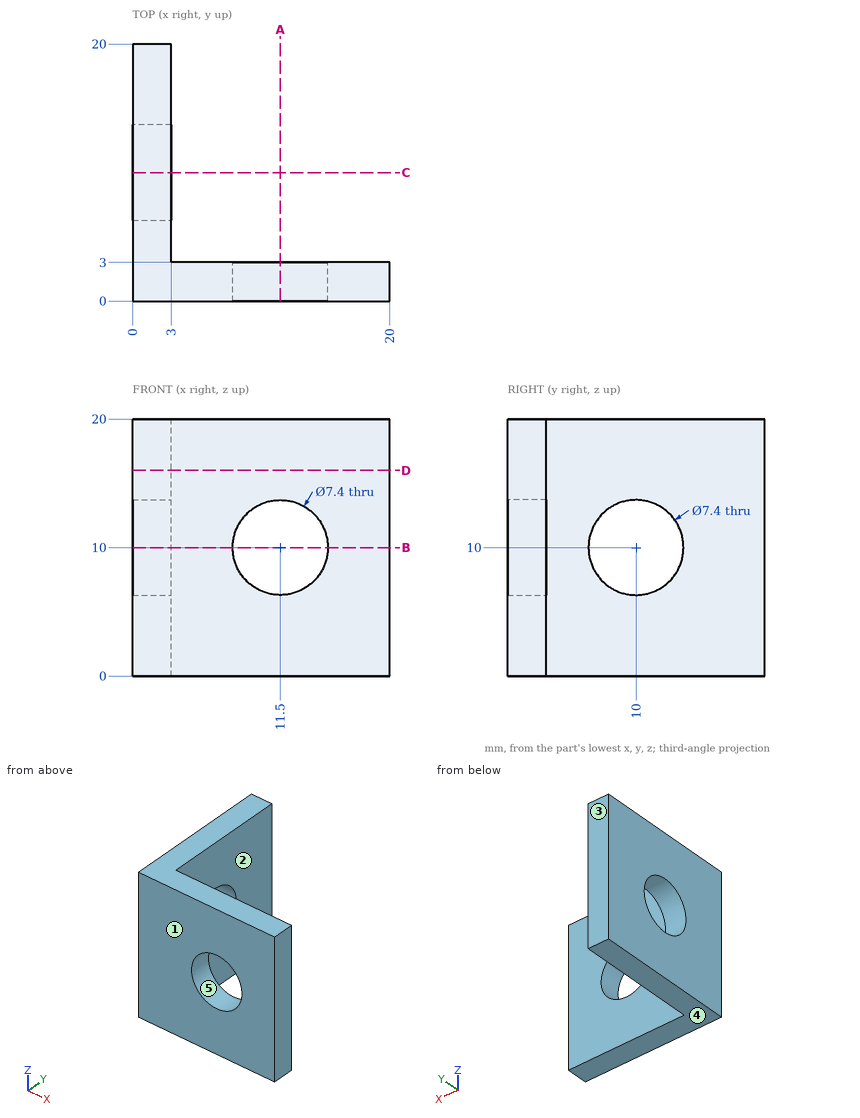
Part print with two shaded views. Sizes in mm from the minimum x, y, z corner. A direction names the side the tool comes from. Give positions to 0.01 mm unless a question says otherwise; leave off trailing zeros. Order: outer loops, then holes, each group sorted by start corner. A loop starts at its lowest first (then second) coordinate and runs counter-clockwise, first axis right, second up.
(1) Drill centre lines: L1, parallel to Z at x = 1.45, y = 10; L2, parallel to X at y = 1.75, z = 10; L3, parallel to X at y = 6.5, z = 2.25. Where is each one in solid material? Low to high.
(2) Flat gauge pins, fed straight in: pin 1 (12 mm diameter, centred on x = 16.5, z = 14.5, fed in from -Y); pin 2 (8.5 mm diameter, centred on y = 15, z = 12.5, fed in from +X); pin 3 (6.5 mm diameter, centred on x = 11.5, z = 10, fed in from -Y). Where does each tip first touch, or does it go through?
(3) Saw through at B-B, the plane z = 10. Give the cut face in (x, y), then the cut area to 3 significant figures.
(4) Saw through at D-D, the plane z = 16. Give the cut face in (x, y), then the cut area to 3 significant figures.
(5) Mould opens along Z. For the marked faces 3, 4 and 5 say: released by +Z, released by -Z, zero draft, split by the parting line, or undercut.
(6) Tool access for the marked faces 1 and 2: list every direction of +Z, -Z, +X, -X, +Y, -Y with a clear straight run to the whole face (end or side of a thin tool).
(7) Saw through at A-A, the plane x = 11.5. Give the cut face in (y, z).
Results found:
1. L1: z = 0 to 6.3, 13.7 to 20
1. L2: x = 0 to 7.8, 15.2 to 20
1. L3: x = 0 to 3
2. pin 1: stops at y = 0
2. pin 2: stops at x = 3
2. pin 3: passes through
3. outline: (0, 0) - (7.8, 0) - (7.8, 3) - (3, 3) - (3, 6.3) - (0, 6.3) - close; (0, 13.7) - (3, 13.7) - (3, 20) - (0, 20) - close; (15.2, 0) - (20, 0) - (20, 3) - (15.2, 3) - close
3. area: 66.6 mm2
4. outline: (0, 0) - (20, 0) - (20, 3) - (3, 3) - (3, 20) - (0, 20) - close
4. area: 111 mm2
5. face 3: zero draft
5. face 4: released by -Z
5. face 5: undercut
6. face 1: +Z, -Z, +X, -X, -Y
6. face 2: +Z, -Z, +X, +Y
7. outline: (0, 0) - (3, 0) - (3, 6.3) - (0, 6.3) - close; (0, 13.7) - (3, 13.7) - (3, 20) - (0, 20) - close
